```python
from build123d import *

# Parameters (mm, degrees)
SKETCH1_W                      = 20
SKETCH1_H                      = 70
BOSS_EXTRUDE1_DEPTH            = 30
SKETCH2_W                      = 12
SKETCH2_H                      = 20
CUT_EXTRUDE1_DEPTH             = 51.249378106
FILLET1_R                      = 10
FILLET2_R                      = 5
CUT_EXTRUDE2_DEPTH             = 51.249378275
FILLET3_R                      = 7
FILLET4_R                      = 7
F_4_0_REAMED_HOLE_D            = 4
F_4_0_REAMED_HOLE_DEPTH        = 5
M3X0_5_TAPPED_HOLE1_D          = 2.5
F_4_0_REAMED_HOLE_BOTTOM_D     = 4
F_4_0_REAMED_HOLE_BOTTOM_DEPTH = 5
F_4_0_REAMED_HOLE_BOTTOM_TIP   = 1.201721238
M4X0_7_TAPPED_HOLE1_D          = 3.3
M4X0_7_TAPPED_HOLE1_DEPTH      = 10.1
M4X0_7_TAPPED_HOLE1_TIP        = 0.991420021


with BuildPart() as part:
    # Sketch1 → Boss-Extrude1 (new body)
    with BuildSketch(Plane(origin=(0, 0, 0), x_dir=(0, 0, -1), z_dir=(1, 0, 0))):
        Rectangle(SKETCH1_W, SKETCH1_H)
    extrude(amount=BOSS_EXTRUDE1_DEPTH)

    # Sketch2 → Cut-Extrude1 (cut, through all)
    with BuildSketch(Plane.XY.offset(10)):
        with Locations((24, -25)):
            Rectangle(SKETCH2_W, SKETCH2_H)
    extrude(amount=-CUT_EXTRUDE1_DEPTH, mode=Mode.SUBTRACT)

    # Fillet1
    fillet1_edges = [part.edges().sort_by_distance(p)[0] for p in [
        (18, -15, 0),
    ]]
    fillet(fillet1_edges, radius=FILLET1_R)

    # Fillet2
    fillet2_edges = [part.edges().sort_by_distance(p)[0] for p in [
        (30, 35, 0),
        (30, -15, 0),
    ]]
    fillet(fillet2_edges, radius=FILLET2_R)

    # Sketch6 → Cut-Extrude2 (cut, through all)
    with BuildSketch(Plane.XY.offset(10)):
        Polygon((0, 30), (25, 30), (25, -10), (8, -10), (8, -25), (0, -25), align=None)
    extrude(amount=-CUT_EXTRUDE2_DEPTH, mode=Mode.SUBTRACT)

    # Fillet3
    fillet3_edges = [part.edges().sort_by_distance(p)[0] for p in [
        (25, 30, 0),
        (25, -10, 0),
        (8, -25, 0),
    ]]
    fillet(fillet3_edges, radius=FILLET3_R)

    # Fillet4
    fillet4_edges = [part.edges().sort_by_distance(p)[0] for p in [
        (8, -10, 0),
    ]]
    fillet(fillet4_edges, radius=FILLET4_R)

    # Ø4.0 Reamed hole
    with Locations(Plane(origin=(0, 35, 0), x_dir=(1, 0, 0), z_dir=(0, 1, 0))):
        with Locations((5, -4), (5, 4), (13, 4), (13, -4)):
            Hole(F_4_0_REAMED_HOLE_D / 2, depth=F_4_0_REAMED_HOLE_DEPTH)

    # M3x0.5 Tapped Hole1 (through all)
    with Locations(Plane(origin=(0, -35, 0), x_dir=(-1, 0, 0), z_dir=(0, -1, 0))):
        with Locations((-5, -4), (-13, -4), (-5, 4), (-13, 4)):
            Hole(M3X0_5_TAPPED_HOLE1_D / 2)

    # Ø4.0 Reamed hole, bottom
    with Locations(Plane(origin=(0, -35, 0), x_dir=(-1, 0, 0), z_dir=(0, -1, 0))):
        with Locations((-5, -4), (-13, -4), (-13, 4), (-5, 4)):
            Hole(F_4_0_REAMED_HOLE_BOTTOM_D / 2, depth=F_4_0_REAMED_HOLE_BOTTOM_DEPTH)
            with Locations((0, 0, -(F_4_0_REAMED_HOLE_BOTTOM_DEPTH + F_4_0_REAMED_HOLE_BOTTOM_TIP / 2))):  # 118° drill point
                Cone(0, F_4_0_REAMED_HOLE_BOTTOM_D / 2, F_4_0_REAMED_HOLE_BOTTOM_TIP, mode=Mode.SUBTRACT)

    # M4x0.7 Tapped Hole1
    with Locations(Plane(origin=(30, 0, 0), x_dir=(0, 0, -1), z_dir=(1, 0, 0))):
        with Locations((-5, 24), (5, 24), (-5, 9), (5, 9), (-5, -6), (5, -6)):
            Hole(M4X0_7_TAPPED_HOLE1_D / 2, depth=M4X0_7_TAPPED_HOLE1_DEPTH)
            with Locations((0, 0, -(M4X0_7_TAPPED_HOLE1_DEPTH + M4X0_7_TAPPED_HOLE1_TIP / 2))):  # 118° drill point
                Cone(0, M4X0_7_TAPPED_HOLE1_D / 2, M4X0_7_TAPPED_HOLE1_TIP, mode=Mode.SUBTRACT)


solid = part.part
```
Verification items for the finished model (mm, model axes). A direction names the side the tool comes from. Round coordinates to 2 decimals unless told otherwise and drop trailing zeros. Order: outer loops, then holes, each group sorted by start corner. A loop starts at its lowest first (then second) coordinate and runs counter-clockwise, first axis right, second up. Notation, with made-up numbers: (20, -20) - (73, -20) arc R5 ccw to (73, -14) - close; hole circle Ø3 at (-12.5, -32.5). An arc over 180 degrees is marked (long way). Use CSV: the item, a comma, the result in double quotes.
(1) Section check B-B on x = 13. State how many separate pieces and enclosed holes the cut face has, and give its area (3 significant figures).
Entries:
separate pieces,"6"
enclosed holes,"0"
area,"415 mm^2"
(2) Section check D-D on y = 13. Record the boundary of the cut face in (x, z), and give its area (3 significant figures).
Entries:
outline,"(25, -10) - (30, -10) - (30, 10) - (25, 10) - close"
area,"100 mm^2"
(3) Gauge pin test, flat ends, axial feed: pin 1 Ø1.5 at (y, z) = (2.5, -5) entering from -X; pin 2 Ø5 at (y, z) = (-30.5, -4) entering from +X; pin 3 Ø3.5 at (x, z) = (13, -4) entering from +Y. Record the tip position at first contact, or that the pin passes through.
Entries:
pin 1,"x = 25"
pin 2,"x = 18"
pin 3,"y = -10"
(4) Mould release check, pull along X, two halves, no side actions. Record for faces 5 (the face through (18, -30, 0)), 6 (the face through (14.6, 32.5, 5.2)), 7 (the face through (16, -11, -10)), 8 (the face through (0, 33, 0)): released by +X, released by -X, zero draft, split by the parting line, or undercut.
Entries:
face 5,"released by +X"
face 6,"undercut"
face 7,"zero draft"
face 8,"released by -X"
(5) Section check A-A on y = 24. Record the boundary of the cut face in (x, z), and give its area (3 significant figures).
Entries:
outline,"(24.93, -10) - (30, -10) - (30, -6.65) - (24.93, -6.65) - close; (24.93, -3.35) - (30, -3.35) - (30, 3.35) - (24.93, 3.35) - close; (24.93, 6.65) - (30, 6.65) - (30, 10) - (24.93, 10) - close"
area,"68.0 mm^2"
(6) Access from +Z, -Z, +X, -X, +Y, -Y to the whole of each face (thin tool, end or side, straight path). Record for faces 1 (the face through (22.9, -8, -0.1)), 2 (the face through (12.01, -19.66, 4.76)), 3 (the face through (5, 32, -2)), 4 (the face through (11.4, -32.5, 5.2)).
Entries:
face 1,"+Z, -Z, -X"
face 2,"+Y, -Y"
face 3,"+Y"
face 4,"-Y"
(7) Thickness scan on probe 1 along Z at (x, y) = (5, -24.5); probe 2 along Z at (x, y) = (28.5, -6); probe 3 along X at (y, z) = (-27, 4). Record the ranges inside material, lowest first. Write a range as from..to.
Entries:
probe 1,"-10..-5.25, -2.75..2.75, 5.25..10"
probe 2,"-10..-6.65, -3.35..3.35, 6.65..10"
probe 3,"0..3.75, 6.25..11.75, 14.25..18"
(8) Section check C-C on y = -6. Record the boundary of the cut face in (x, z).
Entries:
outline,"(24.32, -10) - (30, -10) - (30, -6.65) - (24.32, -6.65) - close; (24.32, -3.35) - (30, -3.35) - (30, 3.35) - (24.32, 3.35) - close; (24.32, 6.65) - (30, 6.65) - (30, 10) - (24.32, 10) - close"
